Source: CAD feature listing. Evaluate the final solid. Frame: model axes, mm. Face numbers are marked on the shaded views. A direction names the side the tool comes from. Give positions to 0.01 mm unless a question says otherwise; leave off trailing zeros. Loops run counter-clockwise (first coordinate to the right, second up) from the corner with the lowest first, then second, coordinate; pieces in that order, holes last.
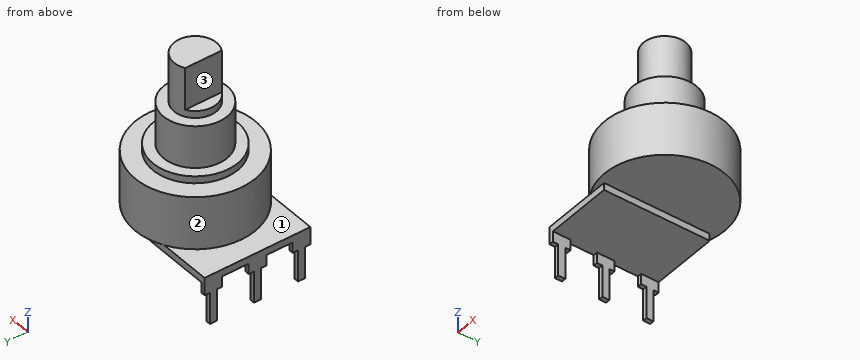
```python
from build123d import *

# Parameters (mm, degrees)
SKETCH_1_R          = 4.5
EXTRUDE_1_DEPTH     = 6
SKETCH_2_R          = 3
EXTRUDE_2_DEPTH     = 7
SKETCH_3_W          = 3.768316072
SKETCH_3_H          = 6.517836593
CUT_EXTRUDE_1_DEPTH = 6
SKETCH_4_R          = 6
EXTRUDE_3_DEPTH     = 1
SKETCH_5_R          = 8.5
EXTRUDE_4_DEPTH     = 7.5
SKETCH_6_W          = 10
SKETCH_6_H          = 15
EXTRUDE_5_DEPTH     = 1
SKETCH_7_W          = 0.6
SKETCH_7_H          = 2.5
EXTRUDE_6_DEPTH     = 6
SKETCH_8_W          = 4.5
SKETCH_8_H          = 0.75
CUT_EXTRUDE_2_DEPTH = 27.645896495


with BuildPart() as part:
    # Эскиз1 → Бобышка-Вытянуть1 (new body)
    with BuildSketch(Plane.XY):
        Circle(SKETCH_1_R)
    extrude(amount=EXTRUDE_1_DEPTH)

    # Эскиз2 → Бобышка-Вытянуть2 (add)
    with BuildSketch(Plane.XY.offset(6)):
        Circle(SKETCH_2_R)
    extrude(amount=EXTRUDE_2_DEPTH)

    # Эскиз3 → Вырез-Вытянуть1 (cut)
    with BuildSketch(Plane.XY.offset(13)):
        with Locations((-3.384158036, 0.355964711)):
            Rectangle(SKETCH_3_W, SKETCH_3_H)
    extrude(amount=-CUT_EXTRUDE_1_DEPTH, mode=Mode.SUBTRACT)

    # Эскиз4 → Бобышка-Вытянуть3 (add)
    with BuildSketch(Plane(origin=(0, 0, 0), x_dir=(-1, 0, 0), z_dir=(0, 0, -1))):
        Circle(SKETCH_4_R)
    extrude(amount=EXTRUDE_3_DEPTH)

    # Эскиз5 → Бобышка-Вытянуть4 (add)
    with BuildSketch(Plane(origin=(0, 0, -1), x_dir=(-1, 0, 0), z_dir=(0, 0, -1))):
        Circle(SKETCH_5_R)
    extrude(amount=EXTRUDE_4_DEPTH)

    # Эскиз6 → Бобышка-Вытянуть5 (add)
    with BuildSketch(Plane(origin=(0, 0, -8.5), x_dir=(-1, 0, 0), z_dir=(0, 0, -1))):
        with Locations((6.437497336, 0)):
            Rectangle(SKETCH_6_W, SKETCH_6_H)
    extrude(amount=EXTRUDE_5_DEPTH)

    # Эскиз7 → Бобышка-Вытянуть6 (add)
    with BuildSketch(Plane(origin=(0, 0, -9.5), x_dir=(-1, 0, 0), z_dir=(0, 0, -1))):
        with Locations((11.137497336, 6.25)):
            Rectangle(SKETCH_7_W, SKETCH_7_H)
        with Locations((11.137497336, 0)):
            Rectangle(SKETCH_7_W, SKETCH_7_H)
        with Locations((11.137497336, -6.25)):
            Rectangle(SKETCH_7_W, SKETCH_7_H)
    extrude(amount=EXTRUDE_6_DEPTH)

    # Эскиз8 → Вырез-Вытянуть2 (cut, through all)
    with BuildSketch(Plane.ZY.offset(11.437497336)):
        with Locations((-13.25, 7.125)):
            Rectangle(SKETCH_8_W, SKETCH_8_H)
        with Locations((-13.25, 5.375)):
            Rectangle(SKETCH_8_W, SKETCH_8_H)
        with Locations((-13.25, 0.875)):
            Rectangle(SKETCH_8_W, SKETCH_8_H)
        with Locations((-13.25, -0.875)):
            Rectangle(SKETCH_8_W, SKETCH_8_H)
        with Locations((-13.25, -5.375)):
            Rectangle(SKETCH_8_W, SKETCH_8_H)
        with Locations((-13.25, -7.125)):
            Rectangle(SKETCH_8_W, SKETCH_8_H)
    extrude(amount=-CUT_EXTRUDE_2_DEPTH, mode=Mode.SUBTRACT)


solid = part.part
```
(1) Section C-C, the plane z = -4.5. Return the cut outline in (x, y), then the cut area to 3 significant figures.
A:
outline: circle Ø17 at (0, 0)
area: 227 mm2
(2) Section A-A, the plane y = 0. Return the cut outline in (x, z), then the cut area to 3 significant figures.
A:
outline: (-11.44, -15.5) - (-10.84, -15.5) - (-10.84, -9.5) - (-1.44, -9.5) - (-1.44, -8.5) - (8.5, -8.5) - (8.5, -1) - (6, -1) - (6, 0) - (4.5, 0) - (4.5, 6) - (3, 6) - (3, 13) - (-1.5, 13) - (-1.5, 7) - (-3, 7) - (-3, 6) - (-4.5, 6) - (-4.5, 0) - (-6, 0) - (-6, -1) - (-8.5, -1) - (-8.5, -8.5) - (-11.44, -8.5) - close
area: 240 mm2
(3) Section D-D, the plane x = -2. Return the cut outline in (y, z), then the cut area to 3 significant figures.
A:
outline: (-8.26, -8.5) - (-7.5, -8.5) - (-7.5, -9.5) - (7.5, -9.5) - (7.5, -8.5) - (8.26, -8.5) - (8.26, -1) - (5.66, -1) - (5.66, 0) - (4.03, 0) - (4.03, 6) - (2.24, 6) - (2.24, 7) - (-2.24, 7) - (-2.24, 6) - (-4.03, 6) - (-4.03, 0) - (-5.66, 0) - (-5.66, -1) - (-8.26, -1) - close
area: 203 mm2
(4) First-contact query: pin 1 (1 mm diameter, centred on x = -8.5, y = -4, fed in from -Z); pin 2 (2 mm diameter, centred on x = -7.5, y = -0.5, fed in from +Z); pin 3 (6 mm diameter, centred on x = -6.5, y = -1.5, fed in from +Z). Flat tips, straight axial feed; report the tip coordinate or a pass-through.
A:
pin 1: stops at z = -9.5
pin 2: stops at z = -1
pin 3: stops at z = 6
(5) Section B-B, the plane x = 0. Return the cut outline in (y, z).
A:
outline: (-8.5, -8.5) - (8.5, -8.5) - (8.5, -1) - (6, -1) - (6, 0) - (4.5, 0) - (4.5, 6) - (3, 6) - (3, 13) - (-3, 13) - (-3, 6) - (-4.5, 6) - (-4.5, 0) - (-6, 0) - (-6, -1) - (-8.5, -1) - close
(6) Reachability of the marked faces 1, 2 and 3 from +Z, -Z, +X, -X, +Y, -Y: full face, straight path, thin tool, end or side. Return the list, or none.
A:
face 1: +Z, -X
face 2: +Z
face 3: +Z, -X, +Y, -Y
(7) Ray query, line 1 along Z through (x, y) = (-1, 5); line 2 along Z through (x, y) = (0, 2.25); line 3 along Y through (x, z) = (-0.25, -4). Return the intervals inside material, ascending.
A:
line 1: z = -8.5 to 0
line 2: z = -8.5 to 13
line 3: y = -8.5 to 8.5
